from build123d import *

# Parameters (mm, degrees)
CHAMFER1_SIZE                                = 1
FILLET1_R                                    = 2
CBORE_FOR_M3_HEX_HEAD_CAP_SCREW1_D           = 3.4
CBORE_FOR_M3_HEX_HEAD_CAP_SCREW1_CBORE_D     = 7
CBORE_FOR_M3_HEX_HEAD_CAP_SCREW1_CBORE_DEPTH = 2
CIRPATTERN1_COUNT                            = 8


with BuildPart() as part:
    # Sketch1 → Revolve1 (revolve)
    with BuildSketch(Plane.XY, mode=Mode.PRIVATE) as revolve1_sk:
        Polygon((7.5, 32), (3.742640687, 32), (0, 28.257359313), (-3.742640687, 32), (-7.5, 32), (-7.5, 17.5), (7.5, 17.5), align=None)
    revolve(revolve1_sk.sketch.rotate(Axis((-33.732241936, 0, 0), (1, 0, 0)), 90), axis=Axis((-33.732241936, 0, 0), (1, 0, 0)))

    # Chamfer1
    chamfer1_edges = [part.edges().sort_by_distance(p)[0] for p in [
        (7.5, 0, -17.5),
        (-7.5, 0, -17.5),
    ]]
    chamfer(chamfer1_edges, length=CHAMFER1_SIZE)

    # Fillet1
    fillet1_edges = [part.edges().sort_by_distance(p)[0] for p in [
        (0, 0, -28.257359313),
    ]]
    fillet(fillet1_edges, radius=FILLET1_R)

    # CBORE for M3 Hex Head Cap Screw1 (through all)
    with Locations(Plane(origin=(7.5, 24, 0), x_dir=(0, 0, 1), z_dir=(1, 0, 0))):
        with Locations((0, 0)):
            cbore_for_m3_hex_head_cap_screw1 = CounterBoreHole(CBORE_FOR_M3_HEX_HEAD_CAP_SCREW1_D / 2, CBORE_FOR_M3_HEX_HEAD_CAP_SCREW1_CBORE_D / 2, CBORE_FOR_M3_HEX_HEAD_CAP_SCREW1_CBORE_DEPTH)

    # CirPattern1: CBORE for M3 Hex Head Cap Screw1 ×8 about axis
    cirpattern1_axis = Axis((0, 0, 0), (1, 0, 0))
    for i in range(1, CIRPATTERN1_COUNT):
        add(cbore_for_m3_hex_head_cap_screw1.rotate(cirpattern1_axis, i * 360 / CIRPATTERN1_COUNT), mode=Mode.SUBTRACT)


solid = part.part
Geometry check sheet. Reference: the model listing, model coordinates, mm. A direction names the side the tool comes from. Round coordinates to 2 decimals unless told otherwise and drop trailing zeros. One line per item, written item: value. Start each with the question number.
(1) Draft check along Y on faces 3 (the flat face through (7.5, 14, -14)), 4 (the flat face through (5.5, -1, -26)), 5 (the cylindrical face through (-5.65, 31.24, -6.94)). Enter one of: +Y half, -Y half, draft (parallel to the pull), parting line (faces both ways), or undercut.
(2) Go/stop test with flat-tipped pins: pin 1 Ø4.5 at (y, z) = (24, 0) entering from +X; pin 2 Ø8 at (y, z) = (-16.97, 16.97) entering from -X; pin 3 Ø1 at (x, y) = (4.5, 16.5) entering from -Z; pin 4 Ø6 at (x, y) = (4, -19.5) entering from +Z. Record where each tip stops, or that it passes through.
(3) Scan lines: line 1 (Y direction, x = -4.25, z = 0); line 2 (Z direction, x = -2.25, y = -16); line 3 (Z direction, x = -1, y = 16). Record each from-to range of solid material in increasing order. Write a range as [from, to].
(4) Access from +Z, -Z, +X, -X, +Y, -Y to the whole of each face (thin tool, end or side, straight path). Record for faces 1 (the cylindrical face through (-1.091, 0.221, -22.314)), 2 (the flat face through (5.5, 15, 17)).
(5) Cross-section at A-A, the plane x = 2.75. Give the number of separate pieces and of enclosed holes in the cut face, and give its area (3 significant figures).
Answer:
1. face 3: draft
1. face 4: undercut
1. face 5: parting line
2. pin 1: x = 5.5
2. pin 2: x = -7.5
2. pin 3: z = -27.71
2. pin 4: z = 27.42
3. line 1: [-32, -25.7], [-22.3, -17.5], [17.5, 22.3], [25.7, 32]
3. line 2: [-25.97, -18.37], [-15.57, -7.09], [7.09, 15.57], [18.37, 25.97]
3. line 3: [-24.61, -18.37], [-15.57, -7.09], [7.09, 15.57], [18.37, 24.61]
4. face 1: +X, -X
4. face 2: +X
5. separate pieces: 1
5. enclosed holes: 9
5. area: 1,990 mm²
